Source: CAD feature listing. Evaluate the final solid. Frame: model axes, mm. Coordinates: 2 decimals unless noted, no trailing zeros. Loops run counter-clockwise (first coordinate to the right, second up) from the corner with the lowest first, then second, coordinate; pieces in that order, holes last. Notation, with made-up numbers: (-15, 8) -> (5, 8) arc R26 ccw to (5, 40) -> close; hole circle Ø1 at (48, 51). An arc over 180 degrees is marked (long way). One line per question, with ' | ' between items. Start each with the question number.
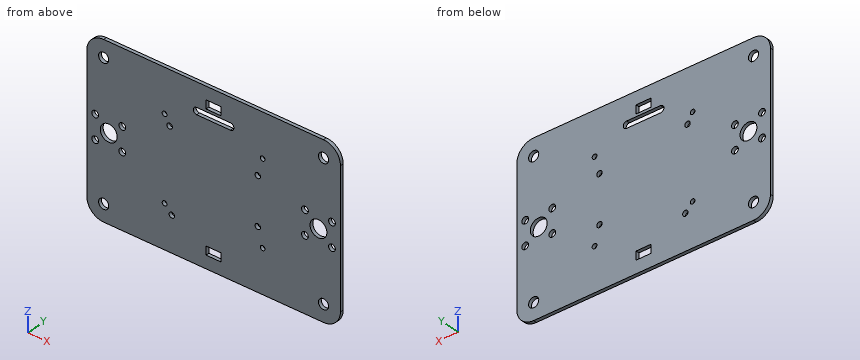
```python
from build123d import *

# Parameters (mm, degrees)
SKETCH1_R           = 1.4
SKETCH1_R_2         = 1.6
SKETCH1_R_3         = 3
SKETCH1_R_4         = 5
SKETCH1_R_5         = 2
SKETCH1_W           = 9
SKETCH1_H           = 5
BOSS_EXTRUDE1_DEPTH = 1


with BuildPart() as part:
    # Sketch1 → Boss-Extrude1 (new, symmetric)
    with BuildSketch(Plane(origin=(0, 0, 0), x_dir=(1, 0, 0), z_dir=(0, 1, 0))):
        with BuildLine():
            Line((-65, -50), (65, -50))
            ThreePointArc((65, -50), (72.071067812, -47.071067812), (75, -40))
            Line((75, -40), (75, 40))
            ThreePointArc((75, 40), (72.071067812, 47.071067812), (65, 50))
            Line((65, 50), (-65, 50))
            ThreePointArc((-65, 50), (-72.071067812, 47.071067812), (-75, 40))
            Line((-75, 40), (-75, -40))
            ThreePointArc((-75, -40), (-72.071067812, -47.071067812), (-65, -50))
        make_face()
        with Locations(Location((-29, 24.5, 0), (0, 0, 270))):
            Circle(SKETCH1_R, mode=Mode.SUBTRACT)
        with Locations(Location((29, 24.5, 0), (0, 0, 270))):
            Circle(SKETCH1_R, mode=Mode.SUBTRACT)
        with Locations(Location((-29, -24.5, 0), (0, 0, 270))):
            Circle(SKETCH1_R, mode=Mode.SUBTRACT)
        with Locations(Location((29, -24.5, 0), (0, 0, 270))):
            Circle(SKETCH1_R, mode=Mode.SUBTRACT)
        with Locations(Location((-24.690715768, 29.15, 0), (0, 0, 270))):
            Circle(SKETCH1_R_2, mode=Mode.SUBTRACT)
        with Locations(Location((-25.990715768, -19.05, 0), (0, 0, 270))):
            Circle(SKETCH1_R_2, mode=Mode.SUBTRACT)
        with Locations(Location((26.109284232, 13.95, 0), (0, 0, 270))):
            Circle(SKETCH1_R_2, mode=Mode.SUBTRACT)
        with Locations(Location((26.109284232, -13.95, 0), (0, 0, 270))):
            Circle(SKETCH1_R_2, mode=Mode.SUBTRACT)
        with Locations(Location((-65, 40, 0), (0, 0, 270))):
            Circle(SKETCH1_R_3, mode=Mode.SUBTRACT)
        with Locations(Location((65, 40, 0), (0, 0, 270))):
            Circle(SKETCH1_R_3, mode=Mode.SUBTRACT)
        with Locations(Location((65, -40, 0), (0, 0, 270))):
            Circle(SKETCH1_R_3, mode=Mode.SUBTRACT)
        with Locations(Location((-65, -40, 0), (0, 0, 270))):
            Circle(SKETCH1_R_3, mode=Mode.SUBTRACT)
        with Locations(Location((-62, 0, 0), (0, 0, 270))):
            Circle(SKETCH1_R_4, mode=Mode.SUBTRACT)
        with Locations(Location((-70, 7, 0), (0, 0, 270))):
            Circle(SKETCH1_R_5, mode=Mode.SUBTRACT)
        with Locations(Location((-54, 7, 0), (0, 0, 270))):
            Circle(SKETCH1_R_5, mode=Mode.SUBTRACT)
        with Locations(Location((-54, -7, 0), (0, 0, 270))):
            Circle(SKETCH1_R_5, mode=Mode.SUBTRACT)
        with Locations(Location((-70, -7, 0), (0, 0, 270))):
            Circle(SKETCH1_R_5, mode=Mode.SUBTRACT)
        with Locations(Location((70, -7, 0), (0, 0, 270))):
            Circle(SKETCH1_R_5, mode=Mode.SUBTRACT)
        with Locations(Location((70, 7, 0), (0, 0, 270))):
            Circle(SKETCH1_R_5, mode=Mode.SUBTRACT)
        with Locations(Location((54, -7, 0), (0, 0, 270))):
            Circle(SKETCH1_R_5, mode=Mode.SUBTRACT)
        with Locations(Location((62, 0, 0), (0, 0, 270))):
            Circle(SKETCH1_R_4, mode=Mode.SUBTRACT)
        with Locations(Location((54, 7, 0), (0, 0, 270))):
            Circle(SKETCH1_R_5, mode=Mode.SUBTRACT)
        with Locations((0, 40)):
            Rectangle(SKETCH1_W, SKETCH1_H, mode=Mode.SUBTRACT)
        with Locations((0, -40)):
            Rectangle(SKETCH1_W, SKETCH1_H, mode=Mode.SUBTRACT)
        with BuildLine():
            Line((-10, -32), (10, -32))
            ThreePointArc((10, -32), (12, -34), (10, -36))
            Line((10, -36), (-10, -36))
            ThreePointArc((-10, -36), (-12, -34), (-10, -32))
        make_face(mode=Mode.SUBTRACT)
    extrude(amount=BOSS_EXTRUDE1_DEPTH, both=True)


solid = part.part
```
(1) Cut plane D-D, the plane z = 34. Return the cut outline in (x, y).
(2) Cut plane B-B, the plane z = 7. Return the cut outline in (x, y).
(3) Ray query, L1, parallel to X at y = -0.3, z = -7; L2, parallel to X at y = -0.2, z = 40; L3, parallel to Z at x = 1, y = 0.2. Return the intervals inside material, ascending.
(4) Cut plane C-C, the plane x = -54. Return the cut outline in (y, z).
(5) Cut plane A-A, the plane z = -13.95. Return the cut outline in (x, y), and give its area (3 significant figures).
Here are the results:
1) outline: (-75, -1) -> (-12, -1) -> (-12, 1) -> (-75, 1) -> close; (12, -1) -> (75, -1) -> (75, 1) -> (12, 1) -> close
2) outline: (-75, -1) -> (-72, -1) -> (-72, 1) -> (-75, 1) -> close; (-68, -1) -> (-56, -1) -> (-56, 1) -> (-68, 1) -> close; (-52, -1) -> (52, -1) -> (52, 1) -> (-52, 1) -> close; (56, -1) -> (68, -1) -> (68, 1) -> (56, 1) -> close; (72, -1) -> (75, -1) -> (75, 1) -> (72, 1) -> close
3) L1: x = -75 to -72, -68 to -56, -52 to 52, 56 to 68, 72 to 75 | L2: x = -75 to -68, -62 to -4.5, 4.5 to 62, 68 to 75 | L3: z = -50 to -42.5, -37.5 to 32, 36 to 37.5, 42.5 to 50
4) outline: (-1, -50) -> (1, -50) -> (1, -9) -> (-1, -9) -> close; (-1, -5) -> (1, -5) -> (1, 5) -> (-1, 5) -> close; (-1, 9) -> (1, 9) -> (1, 50) -> (-1, 50) -> close
5) outline: (-75, -1) -> (24.51, -1) -> (24.51, 1) -> (-75, 1) -> close; (27.71, -1) -> (75, -1) -> (75, 1) -> (27.71, 1) -> close | area: 294 mm2
